Design review of the part built by this model. Coordinates are the model's own, in mm. Face numbers are marked on the shaded views. Coordinates: 2 decimals unless noted, no trailing zeros. Write each loop counter-clockwise with the first axis right and the second up, starting at its lowest first coordinate (ties: lowest second). Pieces come first, ordered by that corner, then holes. Notation, with made-up numbers: M 46,-9 L 76,-9 A18 ccw 76,3 Z; hole C -17.75,86.25 d5. An arc over 180 degrees is marked long. Return JSON: item names as keys, results as strings. Group by question number.
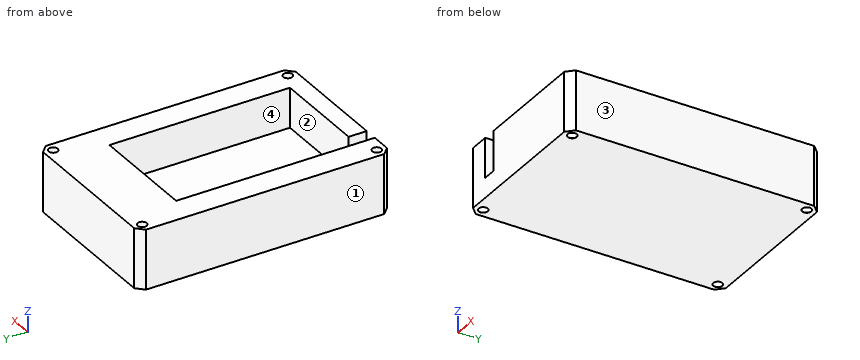
```python
from build123d import *

# Parameters (mm, degrees)
BOSS_EXTRUDE1_DEPTH               = 11
SKETCH1_3_W                       = 30
SKETCH1_3_H                       = 50
SKETCH1_3_W_2                     = 3.611509927
SKETCH1_3_H_2                     = 5
BOSS_EXTRUDE2_DEPTH               = 5.5
TAP_DRILL_FOR_M3_TAP1_D           = 2.5
TAP_DRILL_FOR_M3_TAP1_CSINK_D     = 2.55
TAP_DRILL_FOR_M3_TAP1_CSINK_ANGLE = 90
CHAMFER1_SIZE                     = 2


with BuildPart() as part:
    # Sketch1 → Boss-Extrude1 (new body)
    with BuildSketch(Plane.XY):
        Polygon((-11.388490073, -35), (22.5, -35), (22.5, 35), (-22.5, 35), (-22.5, -35), (-15, -35), (-15, -30), (-15, 20), (15, 20), (15, -30), (-11.388490073, -30), align=None)
    extrude(amount=BOSS_EXTRUDE1_DEPTH)

    # Sketch1_3 → Boss-Extrude2 (add)
    with BuildSketch(Plane.XY):
        Polygon((-11.388490073, -35), (22.5, -35), (22.5, 35), (-22.5, 35), (-22.5, -35), (-15, -35), (-15, -30), (-15, 20), (15, 20), (15, -30), (-11.388490073, -30), align=None)
        with Locations((0, -5)):
            Rectangle(SKETCH1_3_W, SKETCH1_3_H)
        with Locations((-13.194245036, -32.5)):
            Rectangle(SKETCH1_3_W_2, SKETCH1_3_H_2)
    extrude(amount=-BOSS_EXTRUDE2_DEPTH)

    # Tap Drill for M3 Tap1 (through all)
    with Locations(Plane(origin=(0, 0, -5.5), x_dir=(-1, 0, 0), z_dir=(0, 0, -1))):
        with Locations((20, 32.5), (-20, 32.5), (-20, -32.5), (20, -32.5)):
            CounterSinkHole(TAP_DRILL_FOR_M3_TAP1_D / 2, TAP_DRILL_FOR_M3_TAP1_CSINK_D / 2, counter_sink_angle=TAP_DRILL_FOR_M3_TAP1_CSINK_ANGLE)

    # Chamfer1
    chamfer1_edges = [part.edges().sort_by_distance(p)[0] for p in [
        (-22.5, -35, 2.75),
        (-22.5, 35, 2.75),
        (22.5, 35, 2.75),
        (22.5, -35, 2.75),
    ]]
    chamfer(chamfer1_edges, length=CHAMFER1_SIZE)


solid = part.part
```
Item 1: The part is to be moulded in two halves that separate along X. For the marked faces 1, 2, 3 and 4, say which applies: pulls with the +X half, pulls with the -X half, needs draft (parallel to the pull), parting line crosses it, or undercut.
Item 2: For line 1 (Y direction, x = 20, z = -0.5); line 2 (X direction, y = -32.5, z = 7.25); line 3 (X direction, y = 32.5, z = 0), list the stretches that pass through material, from the lowest coordinate up.
Item 3: Add section C-C (y = -2). Write out the cut boundary in (x, z).
Item 4: For pin 1 (2 mm diameter, centred on x = -20, y = -32.5, fed in from +Z); pin 2 (15 mm diameter, centred on x = -7, y = -8.5, fed in from +Z), all flat-tipped, find the tip position at first contact; note any pin that passes through.
Item 5: Add section A-A (z = 3.5). Write out the cut boundary in (x, y).
Item 6: Add section B-B (x = -5). Write out the cut boundary in (y, z).
Geometry check:
{
 "1": {"face 1": "pulls with the -X half", "face 2": "undercut", "face 3": "pulls with the +X half", "face 4": "undercut"},
 "2": {"line 1": "-35 to -33.75, -31.25 to 31.25, 33.75 to 35", "line 2": "-22.5 to -21.25, -18.75 to -15, -11.39 to 18.75, 21.25 to 22.5", "line 3": "-22.5 to -21.25, -18.75 to 18.75, 21.25 to 22.5"},
 "3": {"outline": "M -22.5,-5.5 L 22.5,-5.5 L 22.5,11 L 15,11 L 15,0 L -15,0 L -15,11 L -22.5,11 Z"},
 "4": {"pin 1": "through", "pin 2": "z = 0"},
 "5": {"outline": "M -22.5,-33 L -20.5,-35 L -15,-35 L -15,20 L 15,20 L 15,-30 L -11.39,-30 L -11.39,-35 L 20.5,-35 L 22.5,-33 L 22.5,33 L 20.5,35 L -20.5,35 L -22.5,33 Z; hole C -20,-32.5 d2.5; hole C -20,32.5 d2.5; hole C 20,-32.5 d2.5; hole C 20,32.5 d2.5"},
 "6": {"outline": "M -35,-5.5 L 35,-5.5 L 35,11 L 20,11 L 20,0 L -30,0 L -30,11 L -35,11 Z"}
}
